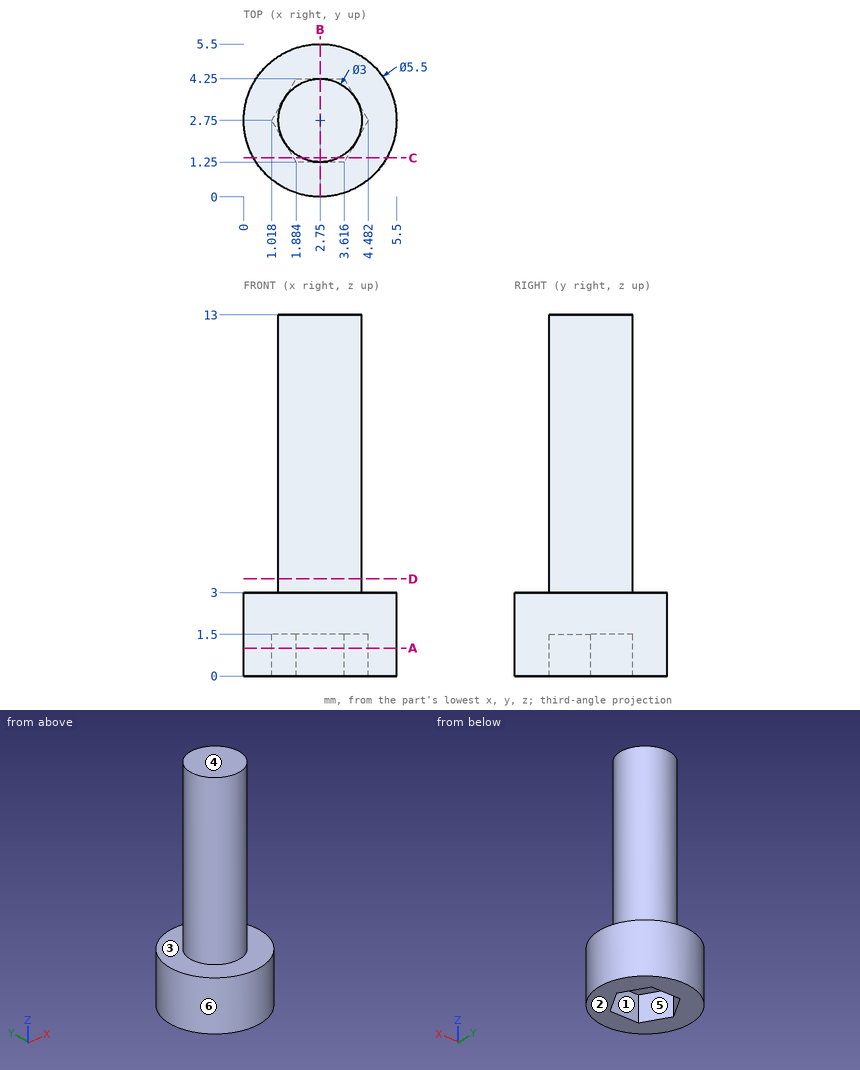
Answer from the drawing. Dimensions are ordinates in mm from the lowest x, y and z of the part. A direction names the side the tool comes from. Give positions to 0.01 mm unless a question says otherwise; leave off trailing zeros. Order: outer loops, then holes, each group sorted by start corner. A loop starts at its lowest first (then second) coordinate and runs counter-clockwise, first axis right, second up. Notation, with made-up numbers: (-16, 56.5) - (-7, 56.5) arc R26 cw to (-7, 94.5) - close; hole circle Ø8 at (54, 43). An arc over 180 degrees is marked (long way). One line per item, written item: value. Start each with the question number.
1. For a pull along X with two mould halves and no side action, classify the marked faces 4, 5 and 6 as released by +X, released by -X, zero draft, split by the parting line, or undercut.
2. Which of the six approach directions +Z, -Z, +X, -X, +Y, -Y give full straight-line access (tool end or side, diameter ignored) to the marked faces 1, 2 and 3?
3. Section B-B, the plane x = 2.75 is taken. Write down the section's boundary in (y, z).
4. This flat-tipped pin is pushed along its axis until it touches: pin 1 Ø1.5 at (x, z) = (1, 5) entering from +Y. Where does it stop, or does it pass through?
5. Section C-C, the plane y = 1.4 is taken. Write down the section's boundary in (x, z).
6. Section A-A, the plane z = 1 is taken. Write down the section's boundary in (x, y), then the cut area to 3 significant figures.
7. Consider line 1 (Z direction, x = 0.3, y = 3.4); line 2 (Z direction, x = 1.35, y = 2.65); line 3 (Y direction, x = 2.85, z = 8.5). Determine where each line is inside the solid, lowest interval first.
8. Section D-D, the plane z = 3.5 is taken. Write down the section's boundary in (x, y).
Filled sheet:
1. face 4: zero draft
1. face 5: undercut
1. face 6: split by the parting line
2. face 1: -Z
2. face 2: -Z, +X, -X, +Y, -Y
2. face 3: +Z
3. outline: (0, 0) - (1.25, 0) - (1.25, 1.5) - (4.25, 1.5) - (4.25, 0) - (5.5, 0) - (5.5, 3) - (4.25, 3) - (4.25, 13) - (1.25, 13) - (1.25, 3) - (0, 3) - close
4. pin 1: y = 3.87
5. outline: (0.35, 0) - (1.8, 0) - (1.8, 1.5) - (3.7, 1.5) - (3.7, 0) - (5.15, 0) - (5.15, 3) - (3.4, 3) - (3.4, 13) - (2.1, 13) - (2.1, 3) - (0.35, 3) - close
6. outline: circle Ø5.5 at (2.75, 2.75); hole (1.02, 2.75) - (1.88, 1.25) - (3.62, 1.25) - (4.48, 2.75) - (3.62, 4.25) - (1.88, 4.25) - close
6. area: 16.0 mm²
7. line 1: 0 to 3
7. line 2: 1.5 to 13
7. line 3: 1.25 to 4.25
8. outline: circle Ø3 at (2.75, 2.75)
